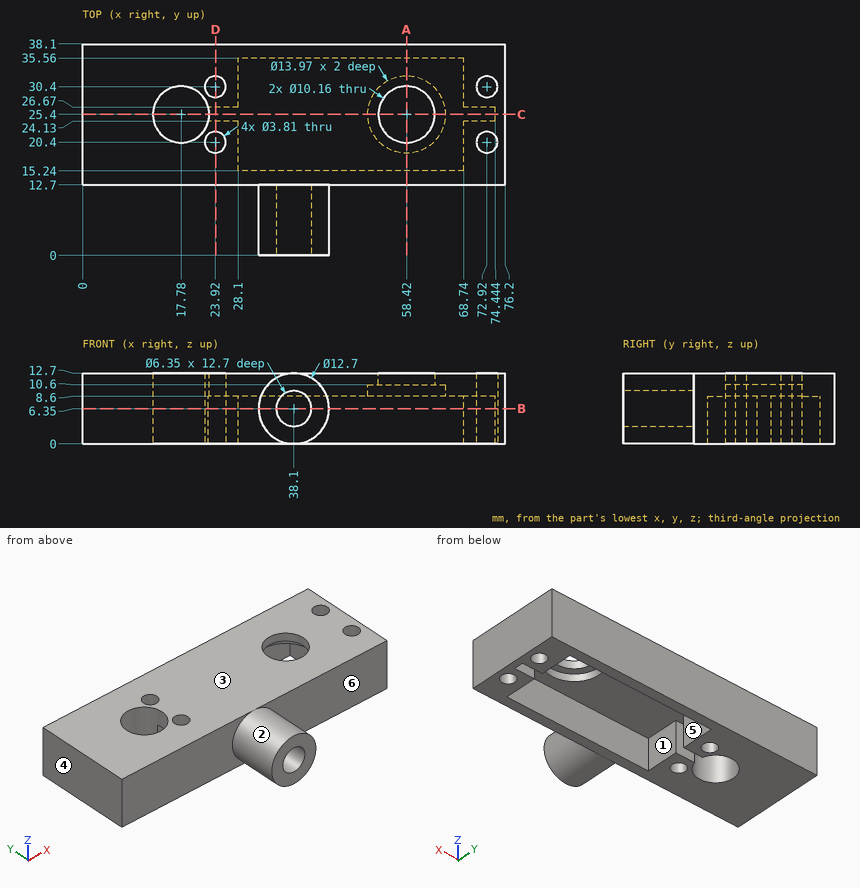
Study the drawing (mm; zero at the part's minimum x, y, z) and answer. A direction names the side the tool comes from. Coordinates: 2 decimals unless noted, no trailing zeros. Order: outer loops, then holes, each group sorted by start corner. A loop starts at its lowest first (then second) coordinate and runs counter-clockwise, first axis right, second up. Notation, with made-up numbers: (66.5, -15) -> (117.5, -15) arc R18 cw to (117.5, -11) -> close; hole circle Ø4 at (46, 76.5). An arc over 180 degrees is marked (long way). Answer in a Markdown table with one row per item. Add a question column.
Item 1: Find section A-A (x = 58.42). Write down the section's boundary in (y, z) (3 decimals).
Item 2: Find section D-D (x = 24). Write down the section's boundary in (y, z), then the cut area to 3 significant figures.
Item 3: Which of the six approach directions +Z, -Z, +X, -X, +Y, -Y give full straight-line access (tool end or side, diameter ignored) to the marked faces 1, 2 and 3?
Item 4: Find section B-B (z = 6.35). State how many separate pieces and enclosed holes the cut face has, then the cut area to 3 significant figures.
Item 5: Find the intervals of material crossed by L1, parallel to Y at x = 71.5, z = 3; L2, parallel to Y at x = 48, z = 3.5; L3, parallel to X at y = 15.5, z = 7.75, in increasing order. Write a range as from..to.
Item 6: Determine the mould class of the marked faces 4, 5 and 6 for opening direction X: +X half, -X half, draft (parallel to the pull), parting line (faces both ways), or undercut.
Item 7: Find section C-C (y = 25.4). Write down the section's boundary in (x, z) (3 decimals).
Item 8: Each of these flat-tipped pins is pushed along its axis until it touches: P1, Ø10, axis at x = 26, y = 7, coming from the -Z side; P2, Ø6, axis at x = 40, y = 28, coming from the -Z side; P3, Ø4.5, axis at x = 71, z = 4.5, coming from the -Y side. Where does it stop, or does it pass through?
Result set:
| question | item | result |
|---|---|---|
| 1 | outline | (12.7, 0) -> (15.24, 0) -> (15.24, 8.6) -> (18.415, 8.6) -> (18.415, 10.6) -> (20.32, 10.6) -> (20.32, 12.7) -> (12.7, 12.7) -> close; (30.48, 10.6) -> (32.385, 10.6) -> (32.385, 8.6) -> (35.56, 8.6) -> (35.56, 0) -> (38.1, 0) -> (38.1, 12.7) -> (30.48, 12.7) -> close |
| 2 | outline | (12.7, 0) -> (18.5, 0) -> (18.5, 12.7) -> (12.7, 12.7) -> close; (22.3, 0) -> (24.13, 0) -> (24.13, 8.6) -> (26.67, 8.6) -> (26.67, 0) -> (28.5, 0) -> (28.5, 12.7) -> (22.3, 12.7) -> close; (32.3, 0) -> (38.1, 0) -> (38.1, 12.7) -> (32.3, 12.7) -> close |
| 2 | area | 204 mm² |
| 3 | face 1 | -Z |
| 3 | face 2 | -Y |
| 3 | face 3 | +Z, +X, -X, +Y, -Y |
| 4 | separate pieces | 1 |
| 4 | enclosed holes | 5 |
| 4 | area | 1,040 mm² |
| 5 | L1 | y = 12.7..19.13, 21.67..24.13, 26.67..29.13, 31.67..38.1 |
| 5 | L2 | y = 12.7..15.24, 35.56..38.1 |
| 5 | L3 | x = 0..28.1, 68.74..76.2 |
| 6 | face 4 | -X half |
| 6 | face 5 | undercut |
| 6 | face 6 | draft |
| 7 | outline | (0, 0) -> (12.7, 0) -> (12.7, 12.7) -> (0, 12.7) -> close; (22.86, 8.6) -> (51.435, 8.6) -> (51.435, 10.6) -> (53.34, 10.6) -> (53.34, 12.7) -> (22.86, 12.7) -> close; (63.5, 10.6) -> (65.405, 10.6) -> (65.405, 8.6) -> (74.444, 8.6) -> (74.444, 0) -> (76.2, 0) -> (76.2, 12.7) -> (63.5, 12.7) -> close |
| 8 | P1 | passes through |
| 8 | P2 | stops at z = 8.6 |
| 8 | P3 | stops at y = 12.7 |
